Study the drawing (mm; zero at the part's minimum x, y, z) and answer. Round coordinates to 2 decimals unless told otherwise and drop trailing zeros. Loops run counter-clockwise (first coordinate to the right, second up) from the corner with the lowest first, then second, coordinate; pieces in that order, holes last. Notation, with made-up numbers: M -6,8 L 34,8 A23 ccw 34,26 Z; hole C 88.25,0.25 d4. An arc over 180 degrees is marked long. Put each result on its own line as item: value. Start each with the question number.
(1) Straight lines are drawn through the part: line 1 (Z direction, x = 5, y = 0.5); line 2 (X direction, y = 0.95, z = 13.5); line 3 (Z direction, x = 3, y = 0.3). For each, find the intervals that lie inside material, in ascending order.
(2) A flat-ended cylindrical pin translates along its axis: P1, Ø4, axis at x = 5, z = 9.5, coming from the -Y side. Find the tip coordinate at first contact, or state that the pin passes through.
(3) Section B-B, the plane x = 7 is taken. Determine the outline of the cut face in (y, z), then the cut area to 3 significant figures.
(4) Section C-C, the plane y = 1.3 is taken. Determine the outline of the cut face in (x, z), then the cut area to 3 significant figures.
(5) Section D-D, the plane z = 9.5 is taken. Determine the outline of the cut face in (x, y).
(6) Section A-A, the plane z = 15 is taken. Determine the outline of the cut face in (x, y).
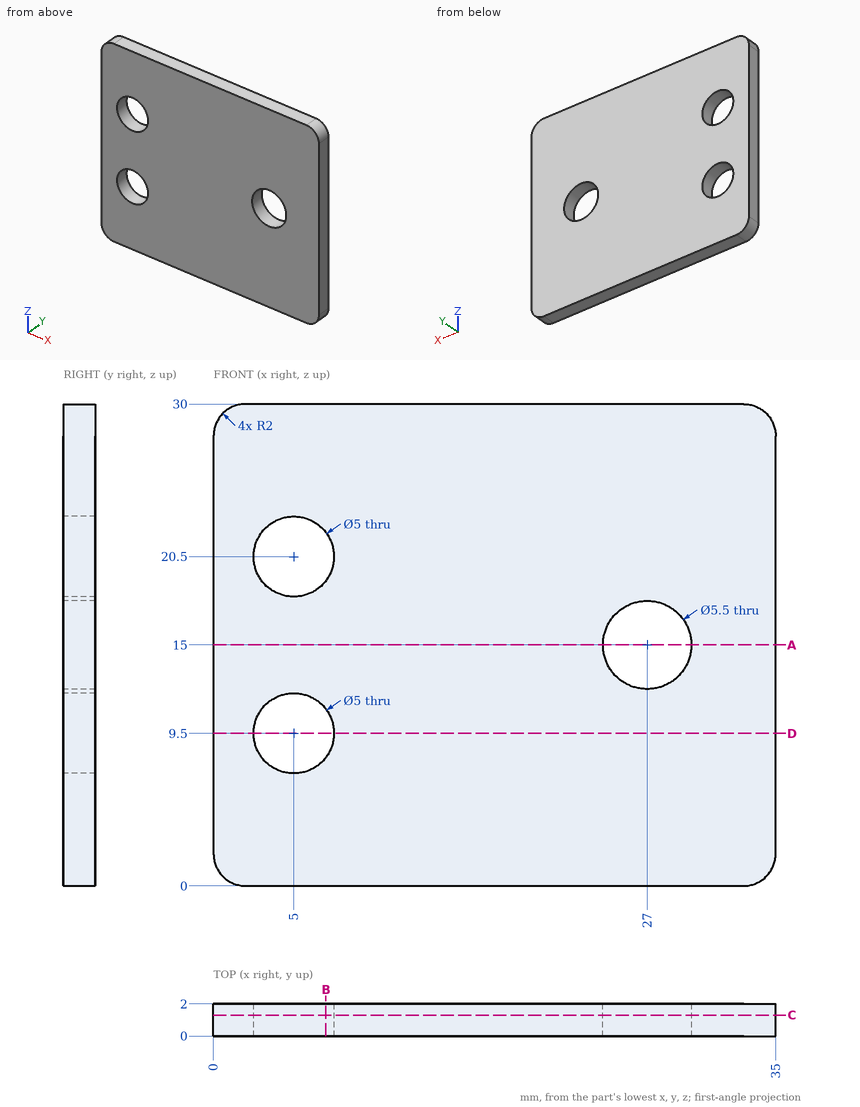
Recorded:
1. line 1: z = 0 to 7, 12 to 18, 23 to 30
1. line 2: x = 0 to 24.7, 29.3 to 35
1. line 3: z = 0 to 8, 11 to 19, 22 to 30
2. P1: passes through
3. outline: M 0,0 L 2,0 L 2,8 L 0,8 Z; M 0,11 L 2,11 L 2,19 L 0,19 Z; M 0,22 L 2,22 L 2,30 L 0,30 Z
3. area: 48.0 mm²
4. outline: M 0,2 A2 ccw 2,0 L 33,0 A2 ccw 35,2 L 35,28 A2 ccw 33,30 L 2,30 A2 ccw 0,28 Z; hole C 5,9.5 d5; hole C 5,20.5 d5; hole C 27,15 d5.5
4. area: 984 mm²
5. outline: M 0,0 L 2.5,0 L 2.5,2 L 0,2 Z; M 7.5,0 L 35,0 L 35,2 L 7.5,2 Z
6. outline: M 0,0 L 24.25,0 L 24.25,2 L 0,2 Z; M 29.75,0 L 35,0 L 35,2 L 29.75,2 Z
